Source: CAD feature listing. Evaluate the final solid. Frame: model axes, mm. Face numbers are marked on the shaded views. A direction names the side the tool comes from. Give positions to 0.01 mm unless a question says otherwise; leave off trailing zeros. Order: outer loops, then holes, each group sorted by start corner. A loop starts at its lowest first (then second) coordinate and runs counter-clockwise, first axis right, second up. Notation, with made-up numbers: (72.25, 12) -> (86.25, 12) arc R14 ccw to (86.25, 26) -> close; hole circle Ø6 at (86.5, 81). An arc over 180 degrees is marked (long way). Use CSV: the item, a comma, the result in double quotes.
```python
from build123d import *

# Parameters (mm, degrees)
F0_R     = 1.5
F1_DEPTH = 25
F2_R     = 2.8
F3_DEPTH = 3
F5_DEPTH = 1.5
F6_SIZE  = 0.25


with BuildPart() as f1:
    # F0 (on Top) → F1 (new body)
    with BuildSketch(Plane.XY):
        Circle(F0_R)
    extrude(amount=F1_DEPTH)

    # F2 (on Top) → F3 (join)
    with BuildSketch(Plane.XY):
        Circle(F2_R)
    extrude(amount=-F3_DEPTH)

    # F4 (on face) → F5 (cut)
    with BuildSketch(Plane(origin=(0, 0, -3), x_dir=(1, 0, 0), z_dir=(0, 0, -1))):
        Polygon((0.446582, -1.372552), (1.411956, -0.299524), (0.965373, 1.073027), (-0.446582, 1.372552), (-1.411956, 0.299524), (-0.965373, -1.073027), align=None)
    extrude(amount=-F5_DEPTH, mode=Mode.SUBTRACT)

    # F6
    f6_edges = [f1.edges().sort_by_distance(p)[0] for p in [
        (-2.8, 0, -3),
        (-1.5, 0, 25),
        (-2.8, 0, 0),
    ]]
    chamfer(f6_edges, length=F6_SIZE)


solid = f1.part
```
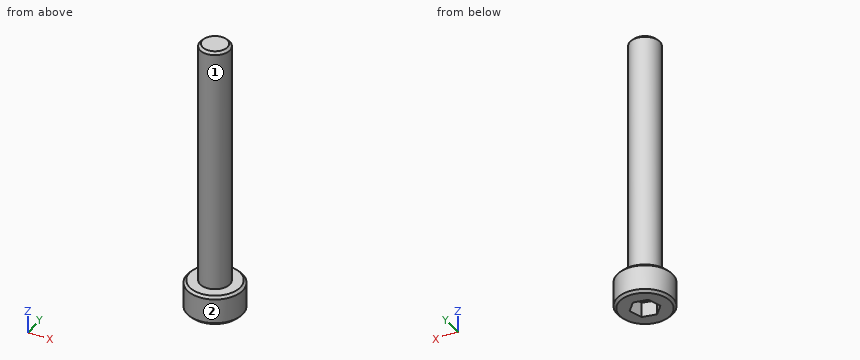
1. Pin query (flat end, axial travel): P1, Ø2, axis at x = -0.5, z = 20.5, coming from the +Y side; P2, Ø1.5, axis at x = 0, z = 6.5, coming from the -Y side; P3, Ø2, axis at y = 0, z = 10.5, coming from the -X side. Return the tip coordinate at first contact, or that it passes through.
Answer below:
P1,"stops at y = 1.5"
P2,"stops at y = -1.5"
P3,"stops at x = -1.5"
2. Section query C-C on z = 23. Return loops of the section in (x, y), plus the area to 3 significant figures.
Answer below:
outline,"circle Ø3 at (0, 0)"
area,"7.07 mm²"
3. Ray query, line 1 along X through (y, z) = (-0.5, 15.5); line 2 along Z through (x, y) = (1.95, 0.4); line 3 along Y through (x, z) = (-0.05, 5.75). Return the intervals inside material, ascending.
Answer below:
line 1,"x = -1.41 to 1.41"
line 2,"z = -3 to 0"
line 3,"y = -1.5 to 1.5"
4. Section query B-B on x = 0. Return loops of the section in (y, z), plus the area to 3 significant figures.
Answer below:
outline,"(-2.8, -2.75) -> (-2.55, -3) -> (-1.28, -3) -> (-1.28, -1.5) -> (1.28, -1.5) -> (1.28, -3) -> (2.55, -3) -> (2.8, -2.75) -> (2.8, -0.25) -> (2.55, 0) -> (1.5, 0) -> (1.5, 24.75) -> (1.25, 25) -> (-1.25, 25) -> (-1.5, 24.75) -> (-1.5, 0) -> (-2.55, 0) -> (-2.8, -0.25) -> close"
area,"87.8 mm²"
5. Section query A-A on y = 0. Return loops of the section in (x, z).
Answer below:
outline,"(-2.8, -2.75) -> (-2.55, -3) -> (-1.31, -3) -> (-1.31, -1.5) -> (1.31, -1.5) -> (1.31, -3) -> (2.55, -3) -> (2.8, -2.75) -> (2.8, -0.25) -> (2.55, 0) -> (1.5, 0) -> (1.5, 24.75) -> (1.25, 25) -> (-1.25, 25) -> (-1.5, 24.75) -> (-1.5, 0) -> (-2.55, 0) -> (-2.8, -0.25) -> close"
6. Access query for the marked faces 1 and 2. Directions: +Z, -Z, +X, -X, +Y, -Y. A direction counts if a zero-diameter tool reaches every point of the face in a straight line with its end or side. Return the directions, or none.
Answer below:
face 1,"+Z"
face 2,"+Z, -Z"
